Autodesk Inventor part; units mm, degrees
ref_plane "YZ Plane" through (0, 0, 0) normal (1, 0, 0) x (0, 1, 0)
ref_plane "XZ Plane" through (0, 0, 0) normal (0, 1, 0) x (-1, 0, 0)
ref_plane "XY Plane" through (0, 0, 0) normal (0, 0, 1) x (1, 0, 0)
sketch "Sketch1" plane through (0, 0, 0) normal (1, 0, 0) x (0, 1, 0)
  line L0 (0, 0) -> (17.2785, 0)
  line L1 (0, -2.5) -> (10, -2.5)
  line L2 (10, -2.5) -> (10, -7.5)
  line L3 (10, -7.5) -> (8.5, -7.5)
  line L4 (8.5, -7.5) -> (8.5, -6)
  line L5 (8.5, -6) -> (1.5, -6)
  line L6 (1.5, -6) -> (1.5, -7.5)
  line L7 (1.5, -7.5) -> (0, -7.5)
  line L8 (0, -7.5) -> (0, -2.5)
  point P0 (5, -2.5)
  dimension "d1" = 5
  dimension "d2" = 15
  dimension "d3" = 12
  dimension "d4" = 7
  dimension "d5" = 1.5
revolve "Revolution1" add sketch "Sketch1" angle 360 about axis through (0, 0, 0) along (0, 1, 0)
properties part number "6mm toothed idler" material "Aluminum 6061"
Design review of the part built by this model. Coordinates are the model's own, in mm. A direction names the side the tool comes from. Coordinates: 2 decimals unless noted, no trailing zeros. Write each loop counter-clockwise with the first axis right and the second up, starting at its lowest first coordinate (ties: lowest second). Pieces come first, ordered by that corner, then holes.
1) To check wall thickness, follow L1, parallel to X at y = 4, z = 0; L2, parallel to Y at x = 5.75, z = 3.5. State the ranges of each line that lie inside material, in increasing order.
2) Machinability: for faces 4 (the flat face through (-6, 1.5, -2)), 5 (the flat face through (-2, 10, 2)), which of the approach directions +Z, -Z, +X, -X, +Y, -Y give a long, thin tool a straight path to every point of the face, cutting with its end or side? Answer none if there is none.
3) Add section C-C (y = 1). Write out the cut boundary in (x, z), plus the area to 3 significant figures.
4) Insertion check: pin 1 (7.5 mm diameter, centred on x = -3.5, z = -2.5, fed in from -Y); pin 2 (1 mm diameter, centred on x = 4.5, y = 2.5, fed in from -Z). Each pin has a flat end and moves straight along its axis. Give the tip position at first contact, or say it passes through.
5) Add section A-A (x = 0). Write out the cut boundary in (y, z).
6) Add section D-D (x = -5.5). Write out the cut boundary in (y, z), plus the area to 3 significant figures.
7) Mouldability with a two-part tool opening along X and no side actions: class faces 1 (the flat face through (-2, 0, 2)), 2 (the cylindrical face through (2.44, 5.07, 0.54)), 3 (the cylindrical face through (0.33, 0.74, 7.493)) as +X half, -X half, draft (parallel to the pull), parting line (faces both ways), or undercut.
8) Add section B-B (z = 0). Write out the cut boundary in (x, y).
Check result:
1. L1: x = -6 to -2.5, 2.5 to 6
1. L2: y = 0 to 1.5, 8.5 to 10
2. face 4: none
2. face 5: +Z, -Z, +X, -X, +Y
3. outline: circle Ø15 at (0, 0); hole circle Ø5 at (0, 0)
3. area: 157 mm2
4. pin 1: stops at y = 0
4. pin 2: stops at z = -4.47
5. outline: (0, -7.5) - (1.5, -7.5) - (1.5, -6) - (8.5, -6) - (8.5, -7.5) - (10, -7.5) - (10, -2.5) - (0, -2.5) - close; (0, 2.5) - (10, 2.5) - (10, 7.5) - (8.5, 7.5) - (8.5, 6) - (1.5, 6) - (1.5, 7.5) - (0, 7.5) - close
6. outline: (0, -5.1) - (1.5, -5.1) - (1.5, -2.4) - (8.5, -2.4) - (8.5, -5.1) - (10, -5.1) - (10, 5.1) - (8.5, 5.1) - (8.5, 2.4) - (1.5, 2.4) - (1.5, 5.1) - (0, 5.1) - close
6. area: 64.2 mm2
7. face 1: draft
7. face 2: undercut
7. face 3: parting line
8. outline: (-7.5, 0) - (-2.5, 0) - (-2.5, 10) - (-7.5, 10) - (-7.5, 8.5) - (-6, 8.5) - (-6, 1.5) - (-7.5, 1.5) - close; (2.5, 0) - (7.5, 0) - (7.5, 1.5) - (6, 1.5) - (6, 8.5) - (7.5, 8.5) - (7.5, 10) - (2.5, 10) - close
